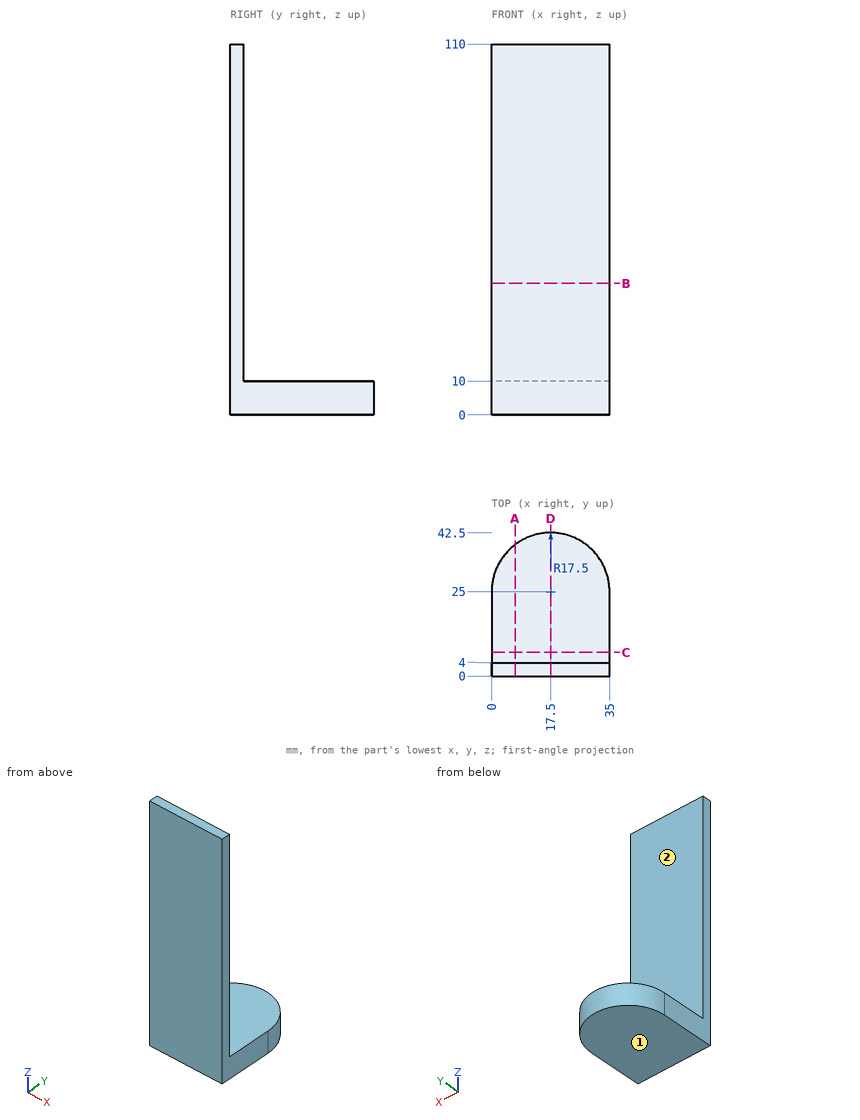
Input: dimensioned drawing with shaded views. Units: mm. Origin: part minimum x, y, z. A direction names the side the tool comes from. Round coordinates to 2 decimals unless told otherwise and drop trailing zeros. Order: outer loops, then holes, each group sorted by start corner. A loop starts at its lowest first (then second) coordinate and runs counter-clockwise, first axis right, second up. Notation, with made-up numbers: M 8,50 L 67,50 A17 cw 67,54 Z; hole C 85,-30.75 d7. An arc over 180 degrees is marked long. Use one line per item in the form item = value. Start each with the question number.
Q1. Cut plane B-B (z = 39). Return loops of the section in (x, y), and give its area (3 significant figures).
Q2. Access query for the marked faces 1 and 2. Directions: +Z, -Z, +X, -X, +Y, -Y. A direction counts if a zero-diameter tool reaches every point of the face in a straight line with its end or side. Return the directions, or none.
Q3. Cut plane A-A (x = 7). Return loops of the section in (y, z), and give its area (3 significant figures).
Q4. Pin query (flat end, axial travel): pin 1 Ø8 at (x, z) = (14.5, 76.5) entering from +Y; pin 2 Ø1 at (x, y) = (21, 18.5) entering from +Z. Return the tip coordinate at first contact, or that it passes through.
Q5. Cut plane C-C (y = 7). Return loops of the section in (x, z).
Q6. Cut plane D-D (x = 17.5). Return loops of the section in (y, z), and give its area (3 significant figures).
Q7. Material intervals for line 1 (Y direction, x = 7, z = 69.5); line 2 (Z direction, x = 27.5, y = 17.5), sorted ascending. Write a range as [from, to].
Geometry results:
q1.outline = M 0,0 L 35,0 L 35,4 L 0,4 Z
q1.area = 140 mm^2
q2.face_1 = -Z, +X, -X, +Y, -Y
q2.face_2 = +Z, +X, -X, +Y
q3.outline = M 0,0 L 39,0 L 39,10 L 4,10 L 4,110 L 0,110 Z
q3.area = 790 mm^2
q4.pin_1 = 4
q4.pin_2 = 10
q5.outline = M 0,0 L 35,0 L 35,10 L 0,10 Z
q6.outline = M 0,0 L 42.5,0 L 42.5,10 L 4,10 L 4,110 L 0,110 Z
q6.area = 825 mm^2
q7.line_1 = [0, 4]
q7.line_2 = [0, 10]
